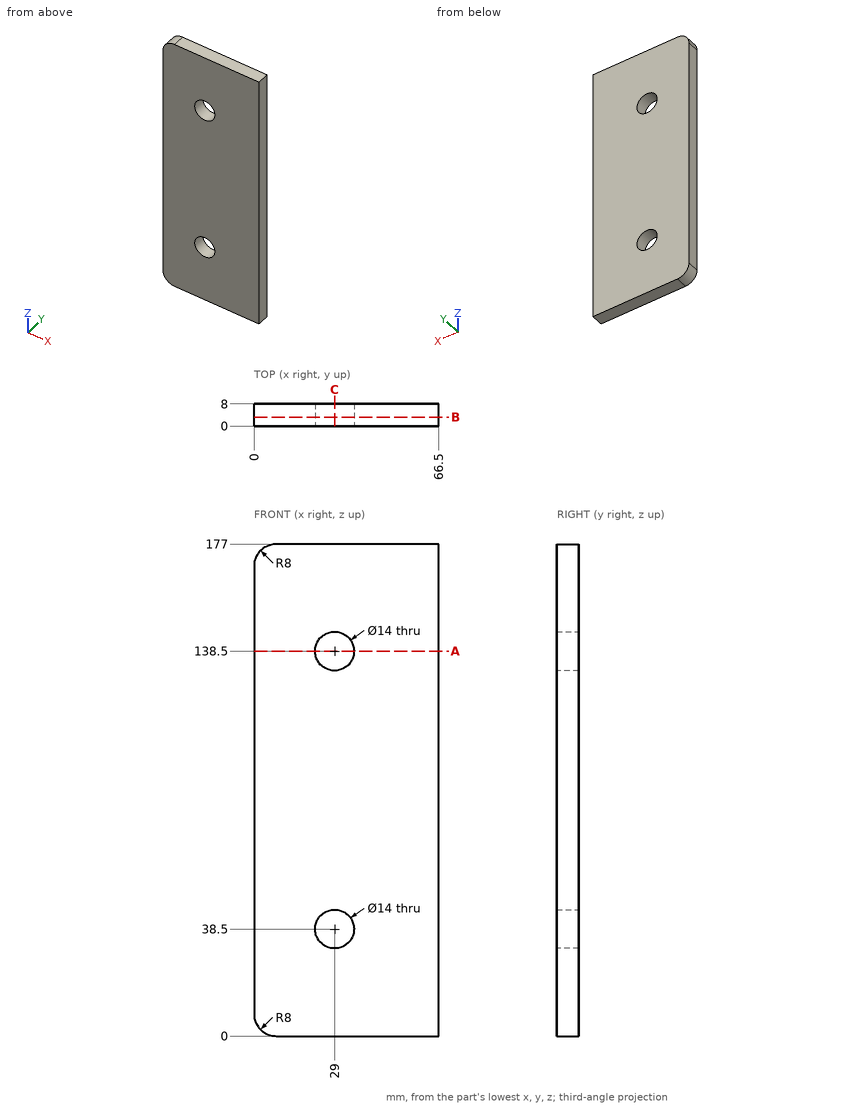
Here's the drawing with two shaded views (mm, measured from the low corner). I have some questions. Give positions to 0.01 mm unless a question says otherwise; leave off trailing zeros. Loops run counter-clockwise (first coordinate to the right, second up) from the corner with the lowest first, then second, coordinate; pieces in that order, holes last. Notation, with made-up numbers: (-36.75, 9) -> (4.25, 9) arc R30 cw to (4.25, 46) -> close; hole circle Ø7 at (-11.5, 54.5). An arc over 180 degrees is marked (long way). One line per item, written item: value.
Q1. Suppose I cut it at C-C on x = 29. Please give me the cut outline in (y, z).
Answers follow:
outline: (0, 0) -> (8, 0) -> (8, 31.5) -> (0, 31.5) -> close; (0, 45.5) -> (8, 45.5) -> (8, 131.5) -> (0, 131.5) -> close; (0, 145.5) -> (8, 145.5) -> (8, 177) -> (0, 177) -> close
Q2. Suppose I cut it at A-A on z = 138.5. Please give me the cut outline in (x, y), then the cut area to 3 significant figures.
Answers follow:
outline: (0, 0) -> (22, 0) -> (22, 8) -> (0, 8) -> close; (36, 0) -> (66.5, 0) -> (66.5, 8) -> (36, 8) -> close
area: 420 mm^2
Q3. Suppose I cut it at B-B on y = 3.25. Please give me the cut outline in (x, z).
Answers follow:
outline: (0, 8) arc R8 ccw to (8, 0) -> (66.5, 0) -> (66.5, 177) -> (8, 177) arc R8 ccw to (0, 169) -> close; hole circle Ø14 at (29, 38.5); hole circle Ø14 at (29, 138.5)
Q4. If I drill on line 1 along X through (y, z) = (4, 38.5); line 2 along X through (y, z) = (3.25, 33); line 3 along Z through (x, y) = (4, 5), over which ranges is the centre line in solid material (lowest first)?
Answers follow:
line 1: 0 to 22, 36 to 66.5
line 2: 0 to 24.67, 33.33 to 66.5
line 3: 1.07 to 175.93
